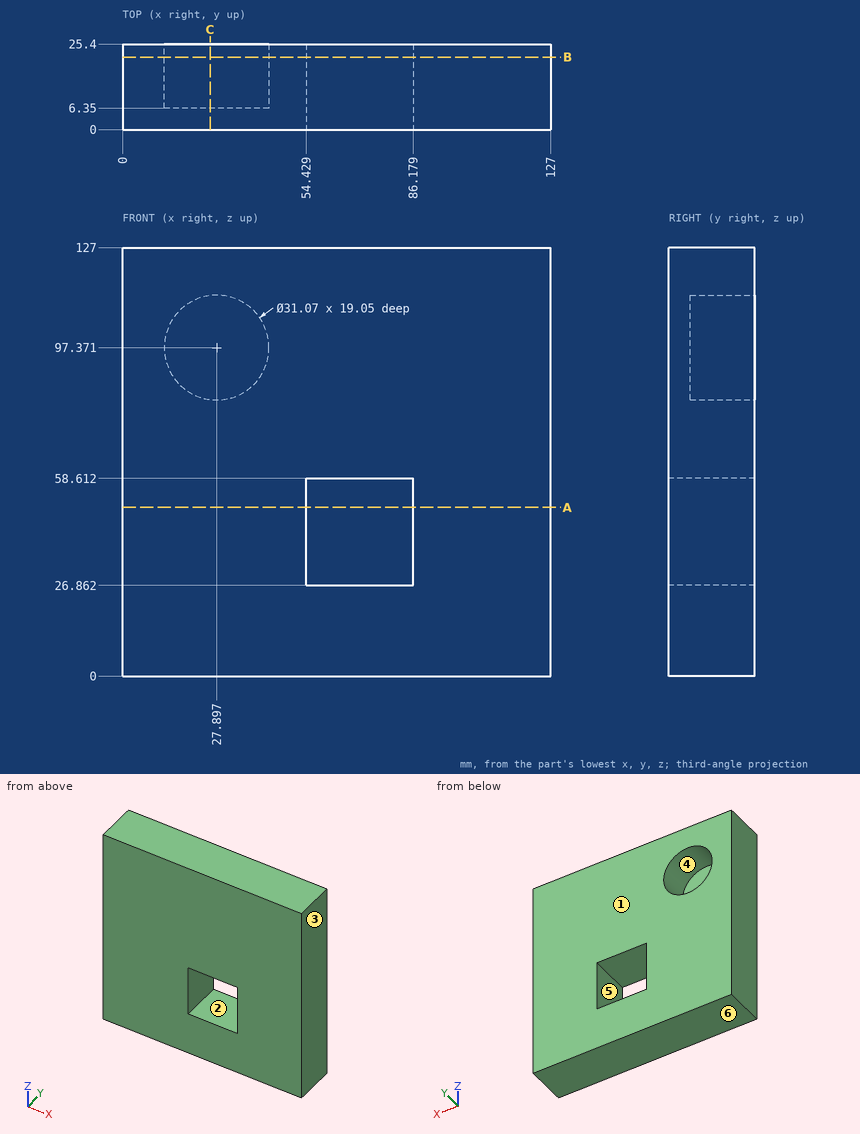
Design review of the part shown in the three views and the two pictorial views. Dimensions are in mm from the part's minimum x, y and z. A direction names the side the tool comes from. Coordinates: 2 decimals unless noted, no trailing zeros. Order: outer loops, then holes, each group sorted by start corner. A loop starts at its lowest first (then second) coordinate and runs counter-clockwise, first axis right, second up.
1) Mouldability with a two-part tool opening along Z and no side actions: class the marked faces 3, 4, 5 and 6 as +Z half, -Z half, draft (parallel to the pull), parting line (faces both ways), or undercut.
2) Wall thickness on line 1 along Z through (x, y) = (69.5, 4); line 2 along X through (y, z) = (3.75, 30.5); line 3 along X through (y, z) = (21.5, 87.5): over which ranges is each line inside the solid? List them lowest first.
3) For the marked faces 1 and 2, list the 3-axis set-ups (+Z, -Z, +X, -X, +Y, -Y) from which the entire face can be reached by the end or side of a thin tool; tool diameter is ignored.
4) Clearance check with a flat-ended pin moving along its axis: pin 1 (15.5 mm diameter, centred on x = 25.5, z = 90, fed in from +Y). State where the tip first meets the part, or that it passes through.
5) Take a section at A-A, the plane z = 50. Give the boundary of the cut face in (x, y), and give its area (3 significant figures).
6) Take a section at B-B, the plane y = 21.5. Give the boundary of the cut face in (x, z) (1 decimal).
7) Take a section at C-C, the plane x = 26. Give the boundary of the cut face in (y, z), and give its area (3 significant figures).
Returned:
1. face 3: draft
1. face 4: undercut
1. face 5: undercut
1. face 6: -Z half
2. line 1: z = 0 to 26.86, 58.61 to 127
2. line 2: x = 0 to 54.43, 86.18 to 127
2. line 3: x = 0 to 15.9, 39.89 to 127
3. face 1: +Z, -Z, +X, -X, +Y
3. face 2: +Y, -Y
4. pin 1: stops at y = 6.35
5. outline: (0, 0) - (54.43, 0) - (54.43, 25.4) - (0, 25.4) - close; (86.18, 0) - (127, 0) - (127, 25.4) - (86.18, 25.4) - close
5. area: 2,420 mm2
6. outline: (0, 0) - (127, 0) - (127, 127) - (0, 127) - close; hole circle Ø31.1 at (27.9, 97.4); hole (54.4, 26.9) - (86.2, 26.9) - (86.2, 58.6) - (54.4, 58.6) - close
7. outline: (0, 0) - (25.4, 0) - (25.4, 81.95) - (6.35, 81.95) - (6.35, 112.79) - (25.4, 112.79) - (25.4, 127) - (0, 127) - close
7. area: 2,640 mm2
